Check sheet for the drawn part. Datum: minimum x, y, z corner. Units: mm. Give positions to 0.01 mm unless a question says otherwise; leave off trailing zeros. Order: outer loops, then holes, each group sorted by start corner. A loop starts at its lowest first (then second) coordinate and runs counter-clockwise, first axis right, second up. Notation, with made-up numbers: M -24,28 L 19,28 A15 cw 19,52 Z; hole C 84,-39.75 d4. An arc over 180 degrees is marked long. Answer as CSV lines item,"result". Start each with the question number.
Q1. Section check D-D, the plane x = 55. Record the boundary of the cut face in (y, z), then the cut area to 3 significant figures.
Q2. Section check B-B, the plane y = 37.5. Record the boundary of the cut face in (x, z).
Q3. Section check A-A, the plane z = 0.45. Record the boundary of the cut face in (x, y).
Q4. Section check C-C, the plane x = 31. Record the boundary of the cut face in (y, z), then the cut area to 3 significant figures.
Q5. Thickness scan on line 1 (Y direction, x = 31, z = 0.2); line 2 (X direction, y = 31.5, z = 0.35); line 3 (X direction, y = 55.5, z = 0.2). Record the ranges inside material, lowest first.
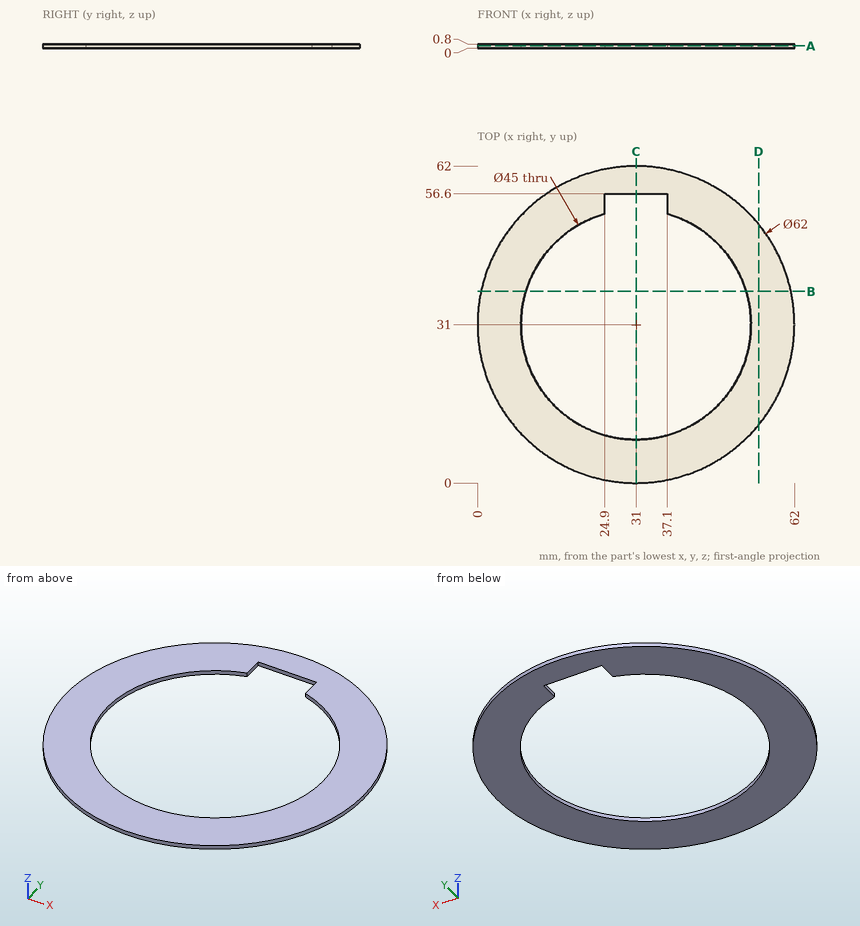
Answer block:
1,outline,"M 11.38,0 L 50.62,0 L 50.62,0.8 L 11.38,0.8 Z"
1,area,"31.4 mm2"
2,outline,"M 0.69,0 L 9.46,0 L 9.46,0.8 L 0.69,0.8 Z; M 52.54,0 L 61.31,0 L 61.31,0.8 L 52.54,0.8 Z"
3,outline,"C 31,31 d62; hole M 24.9,52.66 A22.5 ccw long 37.1,52.66 L 37.1,56.6 L 24.9,56.6 Z"
4,outline,"M 0,0 L 8.5,0 L 8.5,0.8 L 0,0.8 Z; M 56.6,0 L 62,0 L 62,0.8 L 56.6,0.8 Z"
4,area,"11.1 mm2"
5,line 1,"y = 0 to 8.5, 56.6 to 62"
5,line 2,"x = 0 to 8.51, 53.49 to 62"
5,line 3,"x = 12.01 to 24.9, 37.1 to 49.99"
